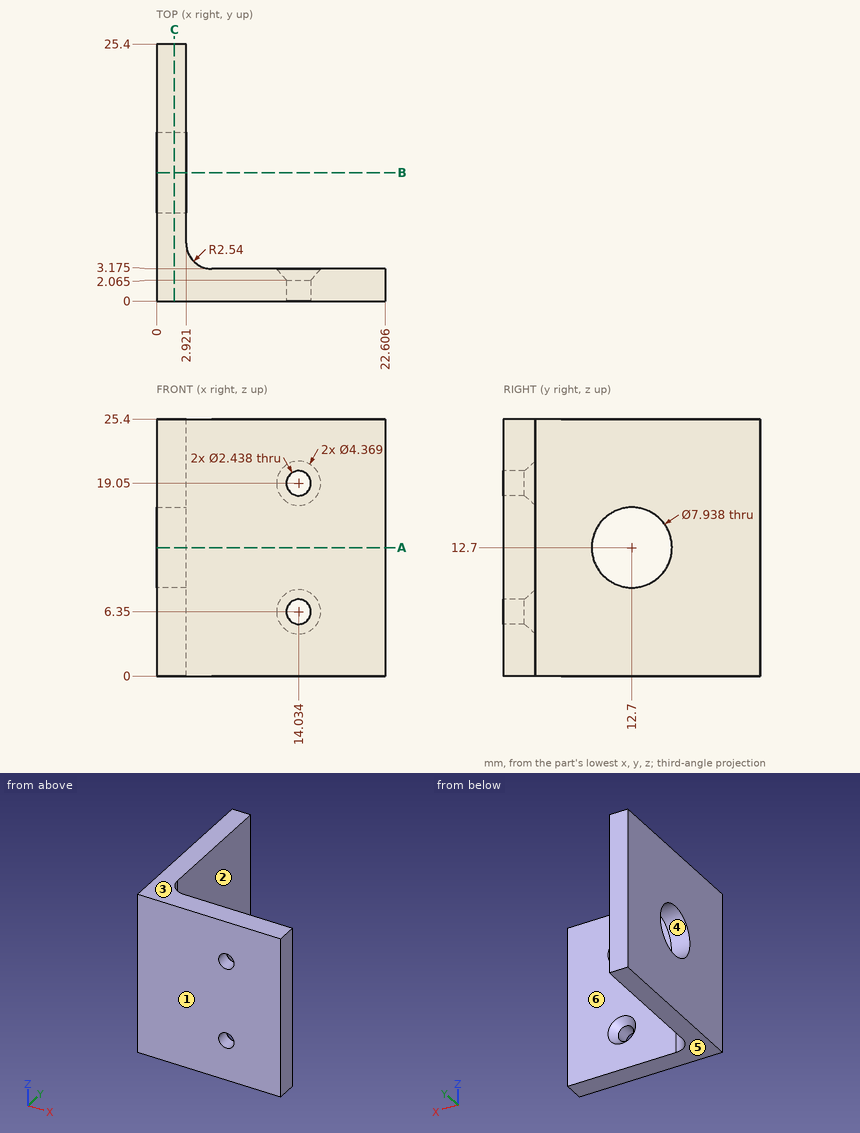
Answer from the drawing. Dimensions are ordinates in mm from the lowest x, y and z of the part. A direction names the side the tool comes from. Coordinates: 2 decimals unless noted, no trailing zeros. Write each loop counter-clockwise with the first axis right and the second up, starting at its lowest first coordinate (ties: lowest second). Pieces come first, ordered by that corner, then holes. Notation, with made-up numbers: M 38.5,56 L 50.5,56 A24 cw 50.5,67 Z; hole C 71.5,9 d2. An arc over 180 degrees is marked long. Put each result on its own line as item: value. Start each with the question number.
1. Consider line 1 (X direction, y = 1.4, z = 19.05) (1 decimal); line 2 (Y direction, x = 1.5, z = 12.7); line 3 (X direction, y = 2, z = 6.5) (1 decimal). Determine where each line is inside the solid, lowest interval first. Write a range as from..to.
2. A cutting plane is placed at A-A on z = 12.7. Write down the section's boundary in (x, y) (1 decimal), then the cut area to 3 significant figures.
3. For a pull along Z with two mould halves and no side action, classify the marked faces 3, 4, 5 and 6 as pulls with the +Z half, pulls with the -Z half, needs draft (parallel to the pull), parting line crosses it, or undercut.
4. Flat-ended cylindrical pins translate along their axes: P1, Ø6, axis at x = 17, z = 4.5, coming from the -Y side; P2, Ø12, axis at y = 20, z = 16.5, coming from the +X side; P3, Ø8.5, axis at x = 11, z = 6.5, coming from the +Y side (1 decimal); P4, Ø4, axis at x = 14.03, z = 6.35, coming from the +Y side (1 decimal). Find the tip coordinate at first contact, or state that the pin passes through.
5. A cutting plane is placed at C-C on x = 1.75. Write down the section's boundary in (y, z), then the cut area to 3 significant figures.
6. Which of the six approach directions +Z, -Z, +X, -X, +Y, -Y give full straight-line access (tool end or side, diameter ignored) to the marked faces 1 and 2?
7. A cutting plane is placed at B-B on y = 12.7. Write down the section's boundary in (x, z).
Resolved:
1. line 1: x = 0..12.8, 15.3..22.6
1. line 2: y = 0..8.73, 16.67..25.4
1. line 3: x = 0..12.8, 15.2..22.6
2. outline: M 0,0 L 22.6,0 L 22.6,3.2 L 5.5,3.2 A2.5 cw 2.9,5.7 L 2.9,8.7 L 0,8.7 Z; M 0,16.7 L 2.9,16.7 L 2.9,25.4 L 0,25.4 Z
2. area: 115 mm2
3. face 3: pulls with the +Z half
3. face 4: undercut
3. face 5: pulls with the -Z half
3. face 6: needs draft
4. P1: stops at y = 0
4. P2: stops at x = 2.92
4. P3: stops at y = 3.2
4. P4: stops at y = 3
5. outline: M 0,0 L 25.4,0 L 25.4,25.4 L 0,25.4 Z; hole C 12.7,12.7 d7.94
5. area: 596 mm2
6. face 1: +Z, -Z, +X, -X, -Y
6. face 2: +Z, -Z, +X, +Y
7. outline: M 0,0 L 2.92,0 L 2.92,8.73 L 0,8.73 Z; M 0,16.67 L 2.92,16.67 L 2.92,25.4 L 0,25.4 Z
